from build123d import *

# Parameters (mm, degrees)
EXTRUDE_1_DEPTH     = 164
SKETCH_3_R          = 1.5
CUT_EXTRUDE_1_DEPTH = 164
SKETCH_4_W          = 2
SKETCH_4_H          = 2
EXTRUDE_2_DEPTH     = 164
SKETCH_5_W          = 0.25
SKETCH_5_H          = 1.5
CUT_EXTRUDE_2_DEPTH = 164
SKETCH_6_W          = 15
SKETCH_6_H          = 50
CUT_EXTRUDE_3_DEPTH = 159
SKETCH_7_W          = 15
SKETCH_7_H          = 1.5
EXTRUDE_3_DEPTH     = 159
SKETCH_8_W          = 3.25
SKETCH_8_H          = 5
EXTRUDE_4_DEPTH     = 15
CUT_EXTRUDE_4_DEPTH = 15
SKETCH_10_R         = 3
CUT_EXTRUDE_5_DEPTH = 2
SKETCH_11_W         = 51.75
SKETCH_11_H         = 2
EXTRUDE_5_DEPTH     = 15
CUT_EXTRUDE_6_DEPTH = 130


with BuildPart() as part:
    # 草图1 → 凸台-拉伸1 (new body)
    with BuildSketch(Plane(origin=(0, 0, 0), x_dir=(1, 0, 0), z_dir=(0, 1, 0))):
        Polygon((0, 0), (0, -65), (3, -65), (3, -50), (18, -50), (18, 0), align=None)
    extrude(amount=EXTRUDE_1_DEPTH)

    # 草图3 → 切除-拉伸1 (cut)
    with BuildSketch(Plane(origin=(0, 164, 0), x_dir=(1, 0, 0), z_dir=(0, 1, 0))):
        with Locations(Location((9, -20, 0), (0, 0, 270))):
            Circle(SKETCH_3_R)
        with Locations(Location((9, -40, 0), (0, 0, 270))):
            Circle(SKETCH_3_R)
    extrude(amount=-CUT_EXTRUDE_1_DEPTH, mode=Mode.SUBTRACT)

    # 草图4 → 凸台-拉伸2 (add)
    with BuildSketch(Plane(origin=(0, 164, 0), x_dir=(1, 0, 0), z_dir=(0, 1, 0))):
        with Locations((-1, -52.5)):
            Rectangle(SKETCH_4_W, SKETCH_4_H)
    extrude(amount=-EXTRUDE_2_DEPTH)

    # 草图5 → 切除-拉伸2 (cut)
    with BuildSketch(Plane.XZ):
        Polygon((-1.75, 51.75), (-2, 51.75), (-2, 51.5), (0, 51.5), (0, 51.75), align=None)
        with Locations((-1.875, 52.5)):
            Rectangle(SKETCH_5_W, SKETCH_5_H)
        Polygon((-2, 53.5), (-2, 53.25), (-1.75, 53.25), (0, 53.25), (0, 53.5), align=None)
    extrude(amount=-CUT_EXTRUDE_2_DEPTH, mode=Mode.SUBTRACT)

    # 草图6 → 切除-拉伸3 (cut)
    with BuildSketch(Plane(origin=(0, 164, 0), x_dir=(1, 0, 0), z_dir=(0, 1, 0))):
        with Locations((10.5, -25)):
            Rectangle(SKETCH_6_W, SKETCH_6_H)
    extrude(amount=-CUT_EXTRUDE_3_DEPTH, mode=Mode.SUBTRACT)

    # 草图7 → 凸台-拉伸3 (add)
    with BuildSketch(Plane(origin=(0, 164, 0), x_dir=(1, 0, 0), z_dir=(0, 1, 0))):
        with Locations((10.5, -52.5)):
            Rectangle(SKETCH_7_W, SKETCH_7_H)
    extrude(amount=-EXTRUDE_3_DEPTH)

    # 草图8 → 凸台-拉伸4 (add)
    with BuildSketch(Plane(origin=(3, 0, 0), x_dir=(0, 0, -1), z_dir=(1, 0, 0))):
        with Locations((-51.625, 2.5)):
            Rectangle(SKETCH_8_W, SKETCH_8_H)
    extrude(amount=EXTRUDE_4_DEPTH)

    # 草图9 → 切除-拉伸4 (cut)
    with BuildSketch(Plane.XY.offset(53.25)):
        Polygon((3, 164), (18, 164), (18, 149), align=None)
    extrude(amount=-CUT_EXTRUDE_4_DEPTH, mode=Mode.SUBTRACT)

    # 草图10 → 切除-拉伸5 (cut)
    with BuildSketch(Plane(origin=(0, 5, 0), x_dir=(1, 0, 0), z_dir=(0, 1, 0))):
        with Locations(Location((9, -20, 0), (0, 0, 270))):
            Circle(SKETCH_10_R)
        with Locations(Location((9, -40, 0), (0, 0, 270))):
            Circle(SKETCH_10_R)
    extrude(amount=-CUT_EXTRUDE_5_DEPTH, mode=Mode.SUBTRACT)

    # 草图11 → 凸台-拉伸5 (add)
    with BuildSketch(Plane(origin=(3, 0, 0), x_dir=(0, 0, -1), z_dir=(1, 0, 0))):
        with Locations((-25.875, 148)):
            Rectangle(SKETCH_11_W, SKETCH_11_H)
        with Locations((-25.875, 138)):
            Rectangle(SKETCH_11_W, SKETCH_11_H)
        with Locations((-25.875, 128)):
            Rectangle(SKETCH_11_W, SKETCH_11_H)
        with Locations((-25.875, 118)):
            Rectangle(SKETCH_11_W, SKETCH_11_H)
        with Locations((-25.875, 108)):
            Rectangle(SKETCH_11_W, SKETCH_11_H)
        with Locations((-25.875, 98)):
            Rectangle(SKETCH_11_W, SKETCH_11_H)
        with Locations((-25.875, 88)):
            Rectangle(SKETCH_11_W, SKETCH_11_H)
        with Locations((-25.875, 78)):
            Rectangle(SKETCH_11_W, SKETCH_11_H)
        with Locations((-25.875, 68)):
            Rectangle(SKETCH_11_W, SKETCH_11_H)
        with Locations((-25.875, 58)):
            Rectangle(SKETCH_11_W, SKETCH_11_H)
        with Locations((-25.875, 48)):
            Rectangle(SKETCH_11_W, SKETCH_11_H)
        with Locations((-25.875, 38)):
            Rectangle(SKETCH_11_W, SKETCH_11_H)
        with Locations((-25.875, 28)):
            Rectangle(SKETCH_11_W, SKETCH_11_H)
    extrude(amount=EXTRUDE_5_DEPTH)

    # 草图12 → 切除-拉伸6 (cut)
    with BuildSketch(Plane(origin=(0, 149, 0), x_dir=(1, 0, 0), z_dir=(0, 1, 0))):
        Polygon((3, 0), (18, -51.75), (18, 0), align=None)
    extrude(amount=-CUT_EXTRUDE_6_DEPTH, mode=Mode.SUBTRACT)


solid = part.part
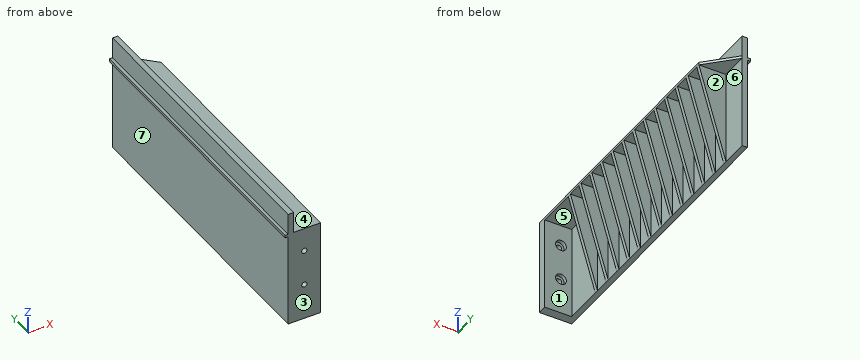
Input: part model. Units: mm. Frame: model coordinates. Face numbers are marked on the shaded views. A direction names the side the tool comes from. Coordinates: 2 decimals unless noted, no trailing zeros. Order: outer loops, then holes, each group sorted by start corner. A loop starts at its lowest first (then second) coordinate and runs counter-clockwise, first axis right, second up. Notation, with made-up numbers: M -37.5,45.5 L -1.5,45.5 A14 ccw -1.5,64.5 Z; hole C 55.5,51 d10. An arc over 180 degrees is marked long. Answer as CSV lines item,"result".
1. Access query for the marked faces 5, 6 and 7. Directions: +Z, -Z, +X, -X, +Y, -Y. A direction counts if a zero-diameter tool reaches every point of the face in a straight line with its end or side. Return the directions, or none.
Reported:
face 5,"-Z, +X"
face 6,"-Z, +X, +Y"
face 7,"-Z, -X, +Y, -Y"
2. Pull-direction query (Y, two-part tool) for the marked faces 1, 2, 3 and 4; classes: released by +Y, released by -Y, zero draft, split by the parting line, or undercut.
Reported:
face 1,"undercut"
face 2,"released by +Y"
face 3,"released by -Y"
face 4,"zero draft"
3. First-contact query: P1, Ø12, axis at y = 147, z = 22.5, coming from the -X side; P2, Ø1.5, axis at x = 14, y = 138.5, coming from the +Z side; P3, Ø1, axis at y = 104.5, z = 25, coming from the +X side. Flat tips, straight axial feed; report the tip coordinate or a pass-through.
Reported:
P1,"x = 0"
P2,"z = 53.25"
P3,"x = 3"
4. Section B-B (x = 9). State how many separate pieces and enclosed holes the cut face has, then the cut area to 3 significant figures.
Reported:
separate pieces,"3"
enclosed holes,"0"
area,"1,260 mm2"
5. Section A-A (y = 145). Return the cut outline in (x, z).
Reported:
outline,"M -1.75,51.75 L 0,51.75 L 0,0 L 3,0 L 3,51.75 L 18,51.75 L 18,53.25 L 3,53.25 L 3,65 L 0,65 L 0,53.25 L -1.75,53.25 Z"
6. Material intervals for line 1 (X direction, y = 2, z = 40); line 2 (Y direction, x = 13, z = 21); line 3 (Z direction, x = 9.25, y = 102.5), sorted ascending. Write a range as from..to.
Reported:
line 1,"0..7.5, 10.5..18"
line 2,"0..5"
line 3,"51.75..53.25"
